```python
from build123d import *

# Parameters (mm, degrees)
SKETCH_1_W          = 20
SKETCH_1_H          = 56
EXTRUDE_1_DEPTH     = 8
SKETCH_2_W          = 4
SKETCH_2_H          = 56
EXTRUDE_2_DEPTH     = 60
FILLET_1_R          = 28
SKETCH_5_R          = 28
EXTRUDE_3_DEPTH     = 2
CUT_EXTRUDE_2_DEPTH = 4.1
SKETCH_6_W          = 20
SKETCH_6_H          = 56
EXTRUDE_4_DEPTH     = 2
SKETCH_7_R          = 10
CUT_EXTRUDE_3_DEPTH = 2
EXTRUDE_5_DEPTH     = 20
SKETCH_3_R          = 4.55
CUT_EXTRUDE_1_DEPTH = 60
SKETCH_9_W          = 15
SKETCH_9_H          = 65
CUT_EXTRUDE_4_DEPTH = 78.768888381


with BuildPart() as part:
    # 스케치1 → 보스-돌출1 (new body)
    with BuildSketch(Plane.XY):
        Rectangle(SKETCH_1_W, SKETCH_1_H)
    extrude(amount=EXTRUDE_1_DEPTH)

    # 스케치2 → 보스-돌출2 (add)
    with BuildSketch(Plane.XY.offset(8)):
        with Locations((8, 0)):
            Rectangle(SKETCH_2_W, SKETCH_2_H)
    extrude(amount=EXTRUDE_2_DEPTH)

    # 필렛1
    fillet_1_edges = [part.edges().sort_by_distance(p)[0] for p in [
        (8, 28, 68),
        (8, -28, 68),
    ]]
    fillet(fillet_1_edges, radius=FILLET_1_R - 0.0001)  # a hair under: the kernel refuses the full size

    # 스케치5 → 보스-돌출3 (add)
    with BuildSketch(Plane(origin=(10, 0, 0), x_dir=(0, 0, -1), z_dir=(1, 0, 0))):
        with Locations(Location((-40, 0, 0), (0, 0, 90))):
            Circle(SKETCH_5_R)
    extrude(amount=EXTRUDE_3_DEPTH)

    # 스케치4 → 컷-돌출2 (cut)
    with BuildSketch(Plane.ZY.offset(-6)):
        with BuildLine():
            Line((35, 16), (35, 19.364916731))
            ThreePointArc((35, 19.364916731), (20, 0), (35, -19.364916731))
            Line((35, -19.364916731), (35, -16))
            Line((35, -16), (45, -16))
            Line((45, -16), (45, -19.364916731))
            ThreePointArc((45, -19.364916731), (55.811388301, -12.247448714), (60, 0))
            ThreePointArc((60, 0), (55.811388301, 12.247448714), (45, 19.364916731))
            Line((45, 19.364916731), (45, 16))
            Line((45, 16), (35, 16))
        make_face()
        with BuildLine():
            ThreePointArc((45, -19.364916731), (40, -20), (35, -19.364916731))
            Line((35, -19.364916731), (35, -24))
            Line((35, -24), (45, -24))
            Line((45, -24), (45, -19.364916731))
        make_face()
        with BuildLine():
            Line((35, -16), (35, -19.364916731))
            ThreePointArc((35, -19.364916731), (40, -20), (45, -19.364916731))
            Line((45, -19.364916731), (45, -16))
            Line((45, -16), (35, -16))
        make_face()
        with BuildLine():
            Line((45, 24), (35, 24))
            Line((35, 24), (35, 19.364916731))
            ThreePointArc((35, 19.364916731), (40, 20), (45, 19.364916731))
            Line((45, 19.364916731), (45, 24))
        make_face()
        with BuildLine():
            ThreePointArc((45, 19.364916731), (40, 20), (35, 19.364916731))
            Line((35, 19.364916731), (35, 16))
            Line((35, 16), (45, 16))
            Line((45, 16), (45, 19.364916731))
        make_face()
    extrude(amount=-CUT_EXTRUDE_2_DEPTH, mode=Mode.SUBTRACT)

    # 스케치6 → 보스-돌출4 (add)
    with BuildSketch(Plane(origin=(10, 0, 0), x_dir=(0, 0, -1), z_dir=(1, 0, 0))):
        with Locations((-10, 0)):
            Rectangle(SKETCH_6_W, SKETCH_6_H)
    extrude(amount=EXTRUDE_4_DEPTH)

    # 스케치7 → 컷-돌출3 (cut)
    with BuildSketch(Plane.ZY.offset(-10.1)):
        with Locations(Location((40, 0, 0), (0, 0, 270))):
            Circle(SKETCH_7_R)
    extrude(amount=-CUT_EXTRUDE_3_DEPTH, mode=Mode.SUBTRACT)

    # 스케치8 → 보스-돌출5 (add)
    with BuildSketch(Plane(origin=(0, 28, 0), x_dir=(1, 0, 0), z_dir=(0, 1, 0))):
        Polygon((-10, -8), (-10, 0), (12, 0), (12, -20), (6, -20), (6, -8), align=None)
    extrude_5 = extrude(amount=EXTRUDE_5_DEPTH)

    # 대칭 복사1: 보스-돌출5 across plane
    add(extrude_5.mirror(Plane.ZX))

    # 스케치3 → 컷-돌출1 (cut)
    with BuildSketch(Plane.XY.offset(8)):
        with Locations((-3, -40.5)):
            Circle(SKETCH_3_R)
        with Locations((-3, 40.5)):
            Circle(SKETCH_3_R)
    extrude(amount=-CUT_EXTRUDE_1_DEPTH, mode=Mode.SUBTRACT)

    # 스케치9 → 컷-돌출4 (cut, through all)
    with BuildSketch(Plane.XY.offset(8)):
        with Locations((-2.5, 0)):
            Rectangle(SKETCH_9_W, SKETCH_9_H)
    extrude(amount=-CUT_EXTRUDE_4_DEPTH, mode=Mode.SUBTRACT)


solid = part.part
```
Source: CAD feature listing. Evaluate the final solid. Frame: model axes, mm. A direction names the side the tool comes from. Give positions to 0.01 mm unless a question says otherwise; leave off trailing zeros. Write each loop counter-clockwise with the first axis right and the second up, starting at its lowest first coordinate (ties: lowest second). Pieces come first, ordered by that corner, then holes.
1. Material intervals for line 1 along Z through (x, y) = (10.9, 0); line 2 along Y through (x, z) = (4.5, 5.5); line 3 along X through (y, z) = (-18.5, 52), sorted ascending.
2. Access query for faces 4 (the face through (8, 24, 40)), 5 (the face through (10, 25, 25)), 6 (the face through (5, 0, 4)), 7 (the face through (8, 28, 30)). Directions: +Z, -Z, +X, -X, +Y, -Y. A direction counts if a zero-diameter tool reaches every point of the face in a straight line with its end or side. Return the directions, or none.
3. Section query A-A (x = 3.25). Return the cut outline in (y, z), then the cut area to 3 significant figures.
4. Section query B-B (z = 37). Return the cut outline in (x, y), then the cut area to 3 significant figures.
5. First-contact query: pin 1 (1 mm diameter, centred on y = -21, z = 25.5, fed in from -X); pin 2 (5 mm diameter, centred on x = 10.5, y = 36.5, fed in from +Z); pin 3 (3.5 mm diameter, centred on x = 8, z = 40, fed in from -Y). Flat tips, straight axial feed; report the tip coordinate or a pass-through.
6. Section query D-D (z = 7). Return the cut outline in (x, y).
7. Pull-direction query (X, two-part tool) for faces 1 (the face through (10, -26, 25)), 2 (the face through (-10, -40, 4)), 3 (the face through (-3.59, 45.01, 4.06)); classes: +X half, -X half, draft (parallel to the pull), parting line (faces both ways), or undercut.
8. Section query C-C (y = -40.5). Return the cut outline in (x, z), then the cut area to 3 significant figures.
Output values:
1. line 1: z = 0 to 30, 50 to 68
1. line 2: y = -48 to -32.5, 32.5 to 48
1. line 3: x = 6 to 12
2. face 4: -X
2. face 5: +X, +Y
2. face 6: +Z, -Z, -X
2. face 7: +Z, +X, -X, +Y
3. outline: (-48, 0) - (-32.5, 0) - (-32.5, 8) - (-48, 8) - close; (32.5, 0) - (48, 0) - (48, 8) - (32.5, 8) - close
3. area: 248 mm2
4. outline: (6, -28) - (10, -28) - (10, -27.84) - (12, -27.84) - (12, -9.54) - (10.1, -9.54) - (10.1, -24) - (6, -24) - close; (6, 24) - (10.1, 24) - (10.1, 9.54) - (12, 9.54) - (12, 27.84) - (10, 27.84) - (10, 28) - (6, 28) - close
4. area: 102 mm2
5. pin 1: stops at x = 6
5. pin 2: stops at z = 20
5. pin 3: stops at y = -28
6. outline: (-10, -48) - (12, -48) - (12, 48) - (-10, 48) - (-10, 32.5) - (5, 32.5) - (5, -32.5) - (-10, -32.5) - close; hole circle Ø9.1 at (-3, -40.5); hole circle Ø9.1 at (-3, 40.5)
7. face 1: +X half
7. face 2: -X half
7. face 3: undercut
8. outline: (-10, 0) - (-7.55, 0) - (-7.55, 8) - (-10, 8) - close; (1.55, 0) - (12, 0) - (12, 20) - (6, 20) - (6, 8) - (1.55, 8) - close
8. area: 175 mm2
